from build123d import *

# Parameters (mm, degrees)
F1_DEPTH      = 5
F2_R          = 1.65
F3_DEPTH      = 3.5
F5_DEPTH      = 5
F5_DEPTH_BACK = 5
F6_R          = 1.6
F6_W          = 12
F6_H          = 23
F7_DEPTH      = 5
F9_DEPTH      = 2.5
F13_ANGLE     = 180
F14_R         = 2
F15_DEPTH     = 25
F17_DEPTH     = 5
F18_R         = 2
F19_DEPTH     = 5.001
F20_R         = 2
F21_DEPTH     = 5.001
F23_DEPTH     = 2


with BuildPart() as f1:
    # F0 (on Top) → F1 (new body)
    with BuildSketch(Plane.XY):
        with BuildLine():
            Line((23, 20), (-23, 20))
            ThreePointArc((-23, 20), (-25.1213203436, 19.1213203436), (-26, 17))
            Line((-26, 17), (-26, -17))
            ThreePointArc((-26, -17), (-25.1213203436, -19.1213203436), (-23, -20))
            Line((-23, -20), (23, -20))
            ThreePointArc((23, -20), (25.1213203436, -19.1213203436), (26, -17))
            Line((26, -17), (26, 17))
            ThreePointArc((26, 17), (25.1213203436, 19.1213203436), (23, 20))
        make_face()
    extrude(amount=F1_DEPTH)

    # F2 (on face) → F3 (cut)
    with BuildSketch(Plane(origin=(0, 0, 0), x_dir=(1, 0, 0), z_dir=(0, 0, -1))):
        Circle(F2_R)
    extrude(amount=-F3_DEPTH, mode=Mode.SUBTRACT)

    # F4 (on Right) → F5 (join, two sides)
    with BuildSketch(Plane.YZ) as f5_sk:
        with BuildLine():
            Line((0, 5), (17, 5))
            Line((17, 5), (4.7831103311, 33.1928223129))
            ThreePointArc((4.7831103311, 33.1928223129), (3.6768840191, 34.5078344182), (2.0304434551, 35))
            Line((2.0304434551, 35), (0, 35))
            Line((0, 35), (0, 5))
        make_face()
        with BuildLine():
            Line((-17, 5), (0, 5))
            Line((0, 5), (0, 35))
            Line((0, 35), (-2.0304434551, 35))
            ThreePointArc((-2.0304434551, 35), (-3.6768840191, 34.5078344182), (-4.7831103311, 33.1928223129))
            Line((-4.7831103311, 33.1928223129), (-17, 5))
        make_face()
    extrude(amount=F5_DEPTH)
    extrude(f5_sk.sketch, amount=-F5_DEPTH_BACK)

    # F6 (on face) → F7 (join)
    with BuildSketch(Plane.YZ.offset(26)):
        with BuildLine():
            Line((17, 0), (17.5, 0))
            Line((17.5, 0), (17.5, 40))
            ThreePointArc((17.5, 40), (16.6213203436, 42.1213203436), (14.5, 43))
            Line((14.5, 43), (-14.5, 43))
            ThreePointArc((-14.5, 43), (-16.6213203436, 42.1213203436), (-17.5, 40))
            Line((-17.5, 40), (-17.5, 0))
            Line((-17.5, 0), (-17, 0))
            Line((-17, 0), (-17, 5))
            Line((-17, 5), (17, 5))
            Line((17, 5), (17, 0))
        make_face()
        with Locations((-9, 24.5)):
            Circle(F6_R, mode=Mode.SUBTRACT)
        with Locations((0, 24.5)):
            Rectangle(F6_W, F6_H, mode=Mode.SUBTRACT)
        with Locations((9, 24.5)):
            Circle(F6_R, mode=Mode.SUBTRACT)
    extrude(amount=-F7_DEPTH)

    # F8 (on face) → F9 (cut)
    with BuildSketch(Plane(origin=(21, 0, 0), x_dir=(0, -1, 0), z_dir=(-1, 0, 0))):
        Polygon((11.8578838325, 26.15), (9, 27.8), (6.1421161675, 26.15), (6.1421161675, 22.85), (9, 21.2), (11.8578838325, 22.85), align=None)
        Polygon((-11.8578838325, 22.85), (-9, 21.2), (-6.1421161675, 22.85), (-6.1421161675, 26.15), (-9, 27.8), (-11.8578838325, 26.15), align=None)
    extrude(amount=-F9_DEPTH, mode=Mode.SUBTRACT)


with BuildPart() as f10_1:
    # F10: copy of F1
    add(f1.part.moved(Location((-47, 0, 0))))


with BuildPart() as f10_1_1:
    # F13: moved
    add(f10_1.part.rotate(Axis((-23.5, 0, 21.4526057243), (0, 0, 1)), F13_ANGLE))


with BuildPart() as f15_tool:
    # F14 (on face) → F15 (new body)
    with BuildSketch(Plane(origin=(-5, 0, 0), x_dir=(0, -1, 0), z_dir=(-1, 0, 0))):
        with Locations((0, 30)):
            Circle(F14_R)
    extrude(amount=-F15_DEPTH)


with BuildPart() as f1_1:
    add(f1.part)

    # F15: cut by f15_tool
    add(f15_tool.part, mode=Mode.SUBTRACT)



with BuildPart() as f10_1_2:
    add(f10_1_1.part)

    # F15: cut by f15_tool
    add(f15_tool.part, mode=Mode.SUBTRACT)


with BuildPart() as f1_2:
    add(f1_1.part)

    add(f10_1_2.part)  # F17 merges F10_1
    # F16 (on face) → F17 (join)
    with BuildSketch(Plane.YZ.offset(-21)):
        with BuildLine():
            Line((17.5, 35), (17.5, 5))
            Line((17.5, 5), (44.2666971773, 36.0169755285))
            ThreePointArc((44.2666971773, 36.0169755285), (45.1678468921, 37.5410467887), (45.4813332936, 39.2836282906))
            Line((45.4813332936, 39.2836282906), (45.4813332936, 49.2836282906))
            ThreePointArc((45.4813332936, 49.2836282906), (40.4813332936, 54.2836282906), (35.4813332936, 49.2836282906))
            Line((35.4813332936, 49.2836282906), (35.4813332936, 42.5987942024))
            Line((35.4813332936, 42.5987942024), (17.5, 35))
        make_face()
    extrude(amount=-F17_DEPTH)

    # F18 (on face) → F19 (cut, through all)
    with BuildSketch(Plane.YZ.offset(-21)):
        with Locations((40.4813332936, 49.2836282906)):
            Circle(F18_R)
    extrude(amount=-F19_DEPTH, mode=Mode.SUBTRACT)

    # F20 (on face) → F21 (cut, through all)
    with BuildSketch(Plane.XY.offset(5)):
        with Locations((-12.5, 0)):
            Circle(F20_R)
        with Locations((12.5, 0)):
            Circle(F20_R)
    extrude(amount=-F21_DEPTH, mode=Mode.SUBTRACT)

    # F22 (on face) → F23 (cut)
    with BuildSketch(Plane(origin=(-5, 0, 0), x_dir=(0, -1, 0), z_dir=(-1, 0, 0))):
        Polygon((-5.0637767885, 25), (-12.4304434551, 8), (12.4304434551, 8), (5.0637767885, 25), align=None)
    extrude(amount=-F23_DEPTH, mode=Mode.SUBTRACT)


solid = f1_2.part
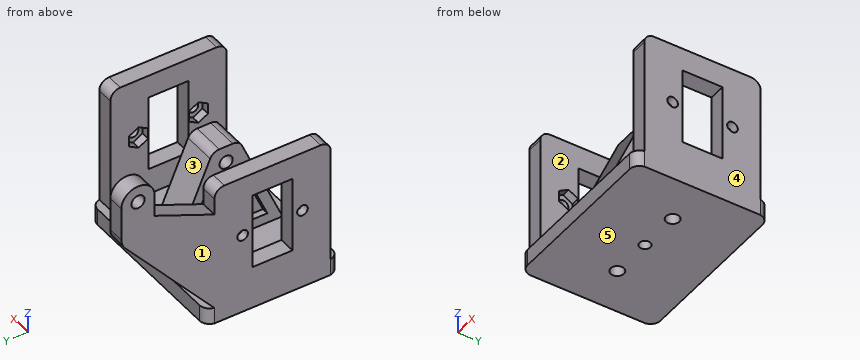
Geometry: final body of the model. Coordinates: model frame, mm. Face numbers are marked on the shaded views. A direction names the side the tool comes from. Give positions to 0.01 mm unless a question says otherwise; leave off trailing zeros. Write each loop counter-clockwise with the first axis right and the second up, starting at its lowest first coordinate (ties: lowest second). Pieces come first, ordered by that corner, then holes.
(1) First-contact query: P1, Ø6, axis at x = 10.5, z = 29, coming from the +Y side; P2, Ø5.5, axis at x = -10, z = 3, coming from the +Y side; P3, Ø2.5, axis at x = -24.5, z = 24.5, coming from the -Y side; P4, Ø10, axis at x = -7, z = 23, coming from the +Y side. Flat tips, straight axial feed; report the tip coordinate or a pass-through.
(2) Access query for the marked faces 1 and 2. Directions: +Z, -Z, +X, -X, +Y, -Y. A direction counts if a zero-diameter tool reaches every point of the face in a straight line with its end or side. Return the directions, or none.
(3) Cut plane C-C, the plane z = 30. Return loops of the section in (x, y).
(4) Cut plane A-A, the plane x = 12.5. Return loops of the section in (y, z).
(5) Cut plane B-B, the plane z = 16.5. Return loops of the section in (x, y).
(6) Mould query, pull axis X, two halves, no side actions, for the marked faces 3, 4 and 5. Classes: released by +X, released by -X, zero draft, split by the parting line, or undercut.
(7) Cut plane D-D, the plane x = 19. Return loops of the section in (y, z).
(8) Ray query, line 1 (X direction, y = -6.5, z = 25.5); line 2 (Z direction, x = -24, y = 9); line 3 (X direction, y = -7.5, z = 34). Return the intervals inside material, ascending.
Values follow:
1. P1: passes through
1. P2: stops at y = 20
1. P3: stops at y = -17.5
1. P4: stops at y = 11.19
2. face 1: +Z, -Z, -X, +Y, -Y
2. face 2: +Z, +Y, -Y
3. outline: (-26, -17.5) - (-21, -17.5) - (-21, -6) - (-26, -6) - close; (-26, 6) - (-21, 6) - (-21, 39.07) - (-26, 39.07) - close; (-5, -6.17) - (5, -6.17) - (5, -2) - (-5, -2) - close; (-5, 2) - (5, 2) - (5, 6.17) - (-5, 6.17) - close; (21, -17.5) - (26, -17.5) - (26, -6) - (21, -6) - close; (21, 6) - (26, 6) - (26, 17.5) - (21, 17.5) - close
4. outline: (-20, 0) - (-2, 0) - (-2, 5) - (-20, 5) - close; (2, 0) - (20, 0) - (20, 5) - (2, 5) - close
5. outline: (-26, -17.5) - (-21, -17.5) - (-21, -6) - (-26, -6) - close; (-26, 6) - (-21, 6) - (-21, 27.42) - (-26, 27.42) - close; (-5, -12.02) - (5, -12.02) - (5, 12.02) - (-5, 12.02) - (-5, 8.75) - (-3, 8.75) - (-3, -8.75) - (-5, -8.75) - close; (21, -17.5) - (26, -17.5) - (26, -6) - (21, -6) - close; (21, 6) - (26, 6) - (26, 17.5) - (21, 17.5) - close
6. face 3: undercut
6. face 4: released by +X
6. face 5: zero draft
7. outline: (-20, 0) - (20, 0) - (20, 5) - (-20, 5) - close
8. line 1: x = -26 to -23.5, -5 to 5, 23.5 to 26
8. line 2: z = 0 to 22.9, 26.1 to 43
8. line 3: x = -26 to -21, 21 to 26
